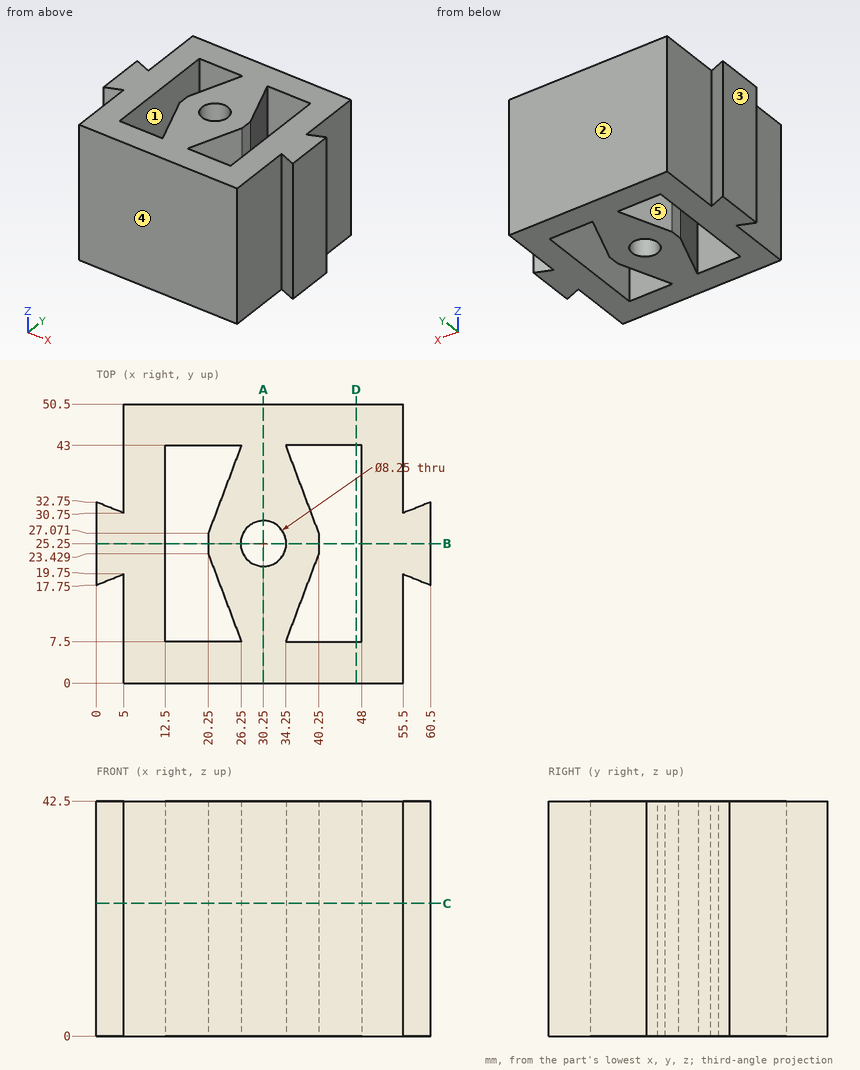
The figure shows three views and two pictorial views of one solid part (mm, origin at its lowest corner). Answer the questions. A direction names the side the tool comes from. Coordinates: 2 decimals unless noted, no trailing zeros. Loops run counter-clockwise (first coordinate to the right, second up) from the corner with the lowest first, then second, coordinate; pieces in that order, holes last. Notation, with made-up numbers: (-34, 3) -> (6, 3) arc R7 ccw to (6, 16) -> close; hole circle Ø7 at (51, 88.5). An arc over 180 degrees is marked (long way). Write item = value, one per line. Start each with the question number.
1) A cutting plane is placed at C-C (z = 24). Give the vertices of the cut face in (x, y) (3 decimals).
2) The mould has two halves that part along X. Classify the marked faces 1, 2 and 3: released by +X, released by -X, zero draft, split by the parting line, or undercut.
3) Given pin 1 Ø7 at (x, z) = (18.5, 26.5) entering from -Y; pin 2 Ø10 at (y, z) = (11, 26) entering from -X; pin 3 Ø7.5 at (x, y) = (30.25, 25.25) entering from +Z; pin 4 Ø6 at (y, z) = (8.5, 25) entering from +X, each flat-ended and moving along its own axis, determine where each tip first touches the part or whether it passes through.
4) Straight lines are drawn through the part: line 1 (X direction, y = 25, z = 17); line 2 (Y direction, x = 47.5, z = 29); line 3 (X direction, y = 34.5, z = 5). For each, find the intervals that lie inside material, in ascending order. Write a range as from..to.
5) A cutting plane is placed at A-A (x = 30.25). Give the vertices of the cut face in (y, z) (3 decimals), then the cut area to 3 significant figures.
6) A tool of negligible diameter and unlimited length cuts with its end or side. For the marked faces 4 and 5, from which of +Z, -Z, +X, -X, +Y, -Y can it reach the whole face along a straight path? Write none if from no direction.
7) A cutting plane is placed at B-B (y = 25.25). Give the vertices of the cut face in (x, z) (3 decimals), then the cut area to 3 significant figures.
8) A cutting plane is placed at D-D (x = 47). Give the vertices of the cut face in (y, z), then the cut area to 4 significant figures.
Responses:
q1.outline = (0, 17.75) -> (5, 19.75) -> (5, 0) -> (55.5, 0) -> (55.5, 19.75) -> (60.5, 17.75) -> (60.5, 32.75) -> (55.5, 30.75) -> (55.5, 50.5) -> (5, 50.5) -> (5, 30.75) -> (0, 32.75) -> close; hole (12.5, 7.5) -> (26.25, 7.5) -> (20.25, 23.429) -> (20.25, 27.071) -> (26.25, 43) -> (12.5, 43) -> close; hole circle Ø8.25 at (30.25, 25.25); hole (34.25, 7.5) -> (48, 7.5) -> (48, 43) -> (34.25, 43) -> (40.25, 27.071) -> (40.25, 23.429) -> close
q2.face_1 = undercut
q2.face_2 = zero draft
q2.face_3 = released by -X
q3.pin_1 = 0
q3.pin_2 = 5
q3.pin_3 = through
q3.pin_4 = 55.5
q4.line_1 = 0..12.5, 20.25..26.13, 34.37..40.25, 48..60.5
q4.line_2 = 0..7.5, 43..50.5
q4.line_3 = 5..12.5, 23.05..37.45, 48..55.5
q5.outline = (0, 0) -> (21.125, 0) -> (21.125, 42.5) -> (0, 42.5) -> close; (29.375, 0) -> (50.5, 0) -> (50.5, 42.5) -> (29.375, 42.5) -> close
q5.area = 1,800 mm²
q6.face_4 = +Z, -Z, +X, -X, -Y
q6.face_5 = +Z, -Z
q7.outline = (0, 0) -> (12.5, 0) -> (12.5, 42.5) -> (0, 42.5) -> close; (20.25, 0) -> (26.125, 0) -> (26.125, 42.5) -> (20.25, 42.5) -> close; (34.375, 0) -> (40.25, 0) -> (40.25, 42.5) -> (34.375, 42.5) -> close; (48, 0) -> (60.5, 0) -> (60.5, 42.5) -> (48, 42.5) -> close
q7.area = 1,560 mm²
q8.outline = (0, 0) -> (7.5, 0) -> (7.5, 42.5) -> (0, 42.5) -> close; (43, 0) -> (50.5, 0) -> (50.5, 42.5) -> (43, 42.5) -> close
q8.area = 637.5 mm²
